For this review, use the dimensioned drawing (mm, ordinates from the lowest corner) and the shaded views. A direction names the side the tool comes from. Coordinates: 2 decimals unless noted, no trailing zeros. Write each loop counter-clockwise with the first axis right and the second up, starting at its lowest first coordinate (ties: lowest second). Pieces come first, ordered by that corner, then holes.
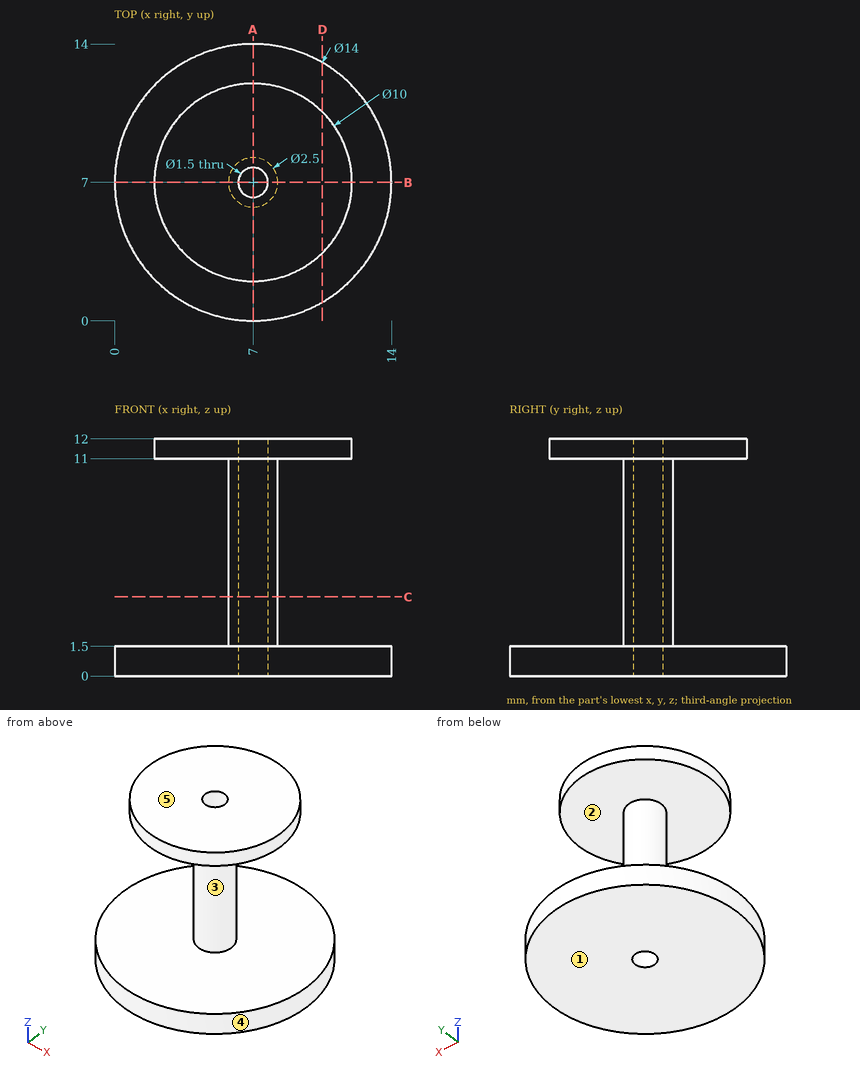
Item 1: To check wall thickness, follow line 1 along Z through (x, y) = (4.25, 6.5); line 2 along Y through (x, z) = (7, 7.5); line 3 along X through (y, z) = (8, 3.75). State the ranges of each line that lie inside material, in increasing order.
Solved:
line 1: z = 0 to 1.5, 11 to 12
line 2: y = 5.75 to 6.25, 7.75 to 8.25
line 3: x = 6.25 to 7.75
Item 2: For pin 1 (3 mm diameter, centred on y = 8, z = 5.5, fed in from +X); pin 2 (0.9 mm diameter, centred on x = 7, y = 7, fed in from +Z); pin 3 (5 mm diameter, centred on x = 9, z = 8, fed in from -Y); pin 4 (1.5 mm diameter, centred on x = 5.5, z = 7, fed in from -Y), all flat-tipped, find the tip position at first contact; note any pin that passes through.
Solved:
pin 1: stops at x = 8.25
pin 2: passes through
pin 3: stops at y = 5.75
pin 4: stops at y = 6
Item 3: Mouldability with a two-part tool opening along Z and no side actions: class the marked faces 3, 4 and 5 as pulls with the +Z half, pulls with the -Z half, needs draft (parallel to the pull), parting line crosses it, or undercut.
Solved:
face 3: undercut
face 4: needs draft
face 5: pulls with the +Z half
Item 4: Take a section at C-C, the plane z = 4. Write out the cut boundary in (x, y), plus the area to 3 significant figures.
Solved:
outline: circle Ø2.5 at (7, 7); hole circle Ø1.5 at (7, 7)
area: 3.14 mm2
Item 5: Machinability: for the marked faces 1 and 2, which of the approach directions +Z, -Z, +X, -X, +Y, -Y give a long, thin tool a straight path to every point of the face, cutting with its end or side? Answer none if there is none.
Solved:
face 1: -Z, +X, -X, +Y, -Y
face 2: none
Item 6: Take a section at A-A, the plane x = 7. Write out the cut boundary in (y, z), plus the area to 4 significant figures.
Solved:
outline: (0, 0) - (6.25, 0) - (6.25, 12) - (2, 12) - (2, 11) - (5.75, 11) - (5.75, 1.5) - (0, 1.5) - close; (7.75, 0) - (14, 0) - (14, 1.5) - (8.25, 1.5) - (8.25, 11) - (12, 11) - (12, 12) - (7.75, 12) - close
area: 36.75 mm2
Item 7: Take a section at D-D, the plane x = 10.5. Write out the cut boundary in (y, z).
Solved:
outline: (0.94, 0) - (13.06, 0) - (13.06, 1.5) - (0.94, 1.5) - close; (3.43, 11) - (10.57, 11) - (10.57, 12) - (3.43, 12) - close
